Geometry: final body of the model. Coordinates: model frame, mm. A direction names the side the tool comes from. Give positions to 0.01 mm unless a question says otherwise; leave off trailing zeros. Loops run counter-clockwise (first coordinate to the right, second up) from the corner with the lowest first, then second, coordinate; pieces in that order, holes last. Notation, with made-up numbers: (33.25, 68) -> (63.25, 68) arc R28 ccw to (63.25, 95) -> close; hole circle Ø8 at (10, -5). An arc over 180 degrees is marked (long way). Answer in a Markdown table with one row per item. Add a question column.
1) Section query B-B (x = 3). Return the cut outline in (y, z).
2) Section query A-A (y = 36). Return the cut outline in (x, z), plus the area to 3 significant figures.
3) First-contact query: P1, Ø2.5, axis at x = 97, y = 28, coming from the -Z side; P2, Ø6, axis at x = 41.5, y = 14, coming from the -Z side; P3, Ø5.5, axis at x = 36.14, y = 12, coming from the +Z side. Flat tips, straight axial feed; report the tip coordinate or a pass-through.
4) Draft query along Y for faces 1 (the flat face through (95, 13, 2.6)), 2 (the flat face through (0, 20, 3)). Return one class per face: +Y half, -Y half, draft (parallel to the pull), parting line (faces both ways), or undercut.
5) Line query: line 1 (Y direction, x = 50, z = 2); line 2 (Y direction, x = 97, z = 5.2); line 3 (X direction, y = 12.5, z = 4.55). Output: solid intervals per line, ascending. Write a range as from..to.
6) Access query for faces 3 (the cylindrical face through (39.146, 26.755, 4.324)), 4 (the cylindrical face through (65.555, 28.075, 1.282)). Directions: +Z, -Z, +X, -X, +Y, -Y. A direction counts if a zero-diameter tool reaches every point of the face in a straight line with its end or side. Return the directions, or none.
7) Section query C-C (z = 1.15). Give the number of separate pieces and of enclosed holes in the cut face, plus the area to 3 significant figures.
```python
from build123d import *

# Parameters (mm, degrees)
SKETCH1_W                                           = 100
SKETCH1_H                                           = 40
BOSS_EXTRUDE1_DEPTH                                 = 6
CBORE_FOR_M3_HEX_SOCKET_HEAD_CAP_SCREW1_D           = 3.4
CBORE_FOR_M3_HEX_SOCKET_HEAD_CAP_SCREW1_CBORE_D     = 6.5
CBORE_FOR_M3_HEX_SOCKET_HEAD_CAP_SCREW1_CBORE_DEPTH = 3.4
CBORE_FOR_M3_HEX_SOCKET_HEAD_CAP_SCREW2_D           = 3.4
CBORE_FOR_M3_HEX_SOCKET_HEAD_CAP_SCREW2_CBORE_D     = 6.5
CBORE_FOR_M3_HEX_SOCKET_HEAD_CAP_SCREW2_CBORE_DEPTH = 3.4


with BuildPart() as part:
    # Sketch1 → Boss-Extrude1 (new body)
    with BuildSketch(Plane.XY):
        with Locations((50, 20)):
            Rectangle(SKETCH1_W, SKETCH1_H)
    extrude(amount=BOSS_EXTRUDE1_DEPTH)

    # CBORE for M3 Hex Socket Head Cap Screw1 (through all)
    with Locations(Plane.XY.offset(6)):
        with Locations((3, 28), (97, 28), (97, 12), (3, 12)):
            CounterBoreHole(CBORE_FOR_M3_HEX_SOCKET_HEAD_CAP_SCREW1_D / 2, CBORE_FOR_M3_HEX_SOCKET_HEAD_CAP_SCREW1_CBORE_D / 2, CBORE_FOR_M3_HEX_SOCKET_HEAD_CAP_SCREW1_CBORE_DEPTH)

    # CBORE for M3 Hex Socket Head Cap Screw2 (through all)
    with Locations(Plane.XY.offset(6)):
        with Locations((36.143593539, 28), (50, 36), (63.856406461, 28), (63.856406461, 12), (50, 4), (36.143593539, 12)):
            CounterBoreHole(CBORE_FOR_M3_HEX_SOCKET_HEAD_CAP_SCREW2_D / 2, CBORE_FOR_M3_HEX_SOCKET_HEAD_CAP_SCREW2_CBORE_D / 2, CBORE_FOR_M3_HEX_SOCKET_HEAD_CAP_SCREW2_CBORE_DEPTH)


solid = part.part
```
Evaluation:
| question | item | result |
|---|---|---|
| 1 | outline | (0, 0) -> (10.3, 0) -> (10.3, 2.6) -> (8.75, 2.6) -> (8.75, 6) -> (0, 6) -> close; (13.7, 0) -> (26.3, 0) -> (26.3, 2.6) -> (24.75, 2.6) -> (24.75, 6) -> (15.25, 6) -> (15.25, 2.6) -> (13.7, 2.6) -> close; (29.7, 0) -> (40, 0) -> (40, 6) -> (31.25, 6) -> (31.25, 2.6) -> (29.7, 2.6) -> close |
| 2 | outline | (0, 0) -> (48.3, 0) -> (48.3, 2.6) -> (46.75, 2.6) -> (46.75, 6) -> (0, 6) -> close; (51.7, 0) -> (100, 0) -> (100, 6) -> (53.25, 6) -> (53.25, 2.6) -> (51.7, 2.6) -> close |
| 2 | area | 569 mm² |
| 3 | P1 | through |
| 3 | P2 | z = 0 |
| 3 | P3 | z = 2.6 |
| 4 | face 1 | undercut |
| 4 | face 2 | draft |
| 5 | line 1 | 0..2.3, 5.7..34.3, 37.7..40 |
| 5 | line 2 | 0..8.75, 15.25..24.75, 31.25..40 |
| 5 | line 3 | 6.21..32.93, 39.35..60.65, 67.07..93.79 |
| 6 | face 3 | +Z |
| 6 | face 4 | +Z, -Z |
| 7 | separate pieces | 1 |
| 7 | enclosed holes | 10 |
| 7 | area | 3,910 mm² |
